Here's how the part is built. I have some questions about the finished solid (model axes, mm). A direction names the side the tool comes from. Give positions to 0.01 mm unless a question says otherwise; leave off trailing zeros. Loops run counter-clockwise (first coordinate to the right, second up) from the corner with the lowest first, then second, coordinate; pieces in that order, holes last. Notation, with made-up numbers: (54, 27.5) - (108, 27.5) arc R23 ccw to (108, 62.5) - close; hole circle Ø5 at (76.25, -15.5). An arc over 180 degrees is marked (long way). Return JSON: item names as keys, results as strings. Group by question number.
(1) If we section it at A-A (y = -4.5): Please give me the cut outline in (x, z), then the cut area to 3 significant figures.
(2) If we mould it in two halves opening along X, with no side actions, what happens to faces 1 (the flat face through (2, -8, 1)), 2 (the cylindrical face through (-2.44, -3.94, 0.54)), 3 (the conical face through (-0.338, 2.812, -1.074)), 4 (the flat face through (0, 0, 0))? For each: released by +X, released by -X, zero draft, split by the parting line, or undercut.
(3) On a 3-axis mill with a long thin cutter (end or side, diameter ignored), from which of +Z, -Z, +X, -X, +Y, -Y can I reach the whole of each face in a straight line? I mean faces 5 (the flat face through (-3, 0, 0)), 6 (the flat face through (11, -8, -13)). Say none if no direction works.
(4) I need wall thicknesses on probe 1 along X at (y, z) = (-2.75, 0); probe 2 along Z at (x, y) = (0.5, -7); probe 3 along Y at (x, z) = (-3.5, 12.5). Which ranges of each line are inside material? Lowest first, please. Write a range as [from, to].
(5) For P1, Ø1, axis at y = -4, z = -8, coming from the -X side; P2, Ø2, axis at x = 11, z = -13.5, coming from the +Y side; P3, Ø6, axis at x = 5.5, y = 0.5, coming from the -Z side, each with a flat end and sliding along its axis, tell me the tip position at first contact or that it passes through.
(6) If we section it at B-B (y = 1): Please give me the cut outline in (x, z), then the cut area to 3 significant figures.
```python
from build123d import *

# Parameters (mm, degrees)
SKETCH2_R           = 18
BOSS_EXTRUDE1_DEPTH = 5
SKETCH3_R           = 17.7
SKETCH3_R_2         = 16.7
BOSS_EXTRUDE2_DEPTH = 3
CUT_EXTRUDE1_START  = -5
SKETCH4_R           = 16.7
CUT_EXTRUDE1_DEPTH  = 5
SKETCH5_R           = 2.5
SKETCH5_R_2         = 2
BOSS_EXTRUDE3_DEPTH = 8


with BuildPart() as part:
    # Sketch1 → Revolve1 (revolve)
    with BuildSketch(Plane(origin=(0, 0, 0), x_dir=(0, 0, -1), z_dir=(1, 0, 0))):
        Polygon((0, 0), (0, 3), (18, 0), align=None)
    revolve(axis=Axis((0, 0, 0), (0, 1, 0)))

    # Sketch2 → Boss-Extrude1 (add)
    with BuildSketch(Plane.XZ):
        with Locations(Location((0, 0, 0), (0, 0, 270))):
            Circle(SKETCH2_R)
    extrude(amount=BOSS_EXTRUDE1_DEPTH)

    # Sketch3 → Boss-Extrude2 (add)
    with BuildSketch(Plane.XZ.offset(5)):
        with Locations(Location((0, 0, 0), (0, 0, 270))):
            Circle(SKETCH3_R)
        with Locations(Location((0, 0, 0), (0, 0, 270))):
            Circle(SKETCH3_R_2, mode=Mode.SUBTRACT)
    extrude(amount=BOSS_EXTRUDE2_DEPTH)

    # Sketch4 → Cut-Extrude1 (cut)
    with BuildSketch(Plane.XZ.offset(5).offset(CUT_EXTRUDE1_START)):
        with Locations(Location((0, 0, 0), (0, 0, 270))):
            Circle(SKETCH4_R)
    extrude(amount=CUT_EXTRUDE1_DEPTH, mode=Mode.SUBTRACT)

    # Sketch5 → Boss-Extrude3 (add)
    with BuildSketch(Plane.XZ):
        with Locations(Location((0, 0, 0), (0, 0, 270))):
            Circle(SKETCH5_R)
        with Locations(Location((0, 0, 0), (0, 0, 270))):
            Circle(SKETCH5_R_2, mode=Mode.SUBTRACT)
    extrude(amount=BOSS_EXTRUDE3_DEPTH)


solid = part.part
```
Values:
{
 "1": {"outline": "circle Ø36 at (0, 0); circle Ø5 at (0, 0); hole circle Ø33.4 at (0, 0); hole circle Ø4 at (0, 0)", "area": "149 mm2"},
 "2": {"face 1": "zero draft", "face 2": "undercut", "face 3": "split by the parting line", "face 4": "undercut"},
 "3": {"face 5": "-Y", "face 6": "+Z, -Z, +X, -X, -Y"},
 "4": {"probe 1": "[-18, -16.7], [-2.5, -2], [2, 2.5], [16.7, 18]", "probe 2": "[-17.69, -16.69], [-2.45, -1.94], [1.94, 2.45], [16.69, 17.69]", "probe 3": "[0, 0.84]"},
 "5": {"P1": "x = -16.36", "P2": "y = 0.26", "P3": "z = -17.82"},
 "6": {"outline": "circle Ø24 at (0, 0)", "area": "452 mm2"}
}
